from build123d import *

# Parameters (mm, degrees)
SKETCH2_R            = 10
BOSS_EXTRUDE1_DEPTH  = 4
BOSS_EXTRUDE2_DEPTH  = 10
FILLET1_R            = 5
M3_CLEARANCE_HOLE1_D = 3.6
FILLET2_R            = 3


with BuildPart() as part:
    # Sketch2 → Boss-Extrude1 (new body)
    with BuildSketch(Plane(origin=(0, 0, 0), x_dir=(1, 0, 0), z_dir=(0, 1, 0))):
        with BuildLine():
            Line((34.142135624, 5), (34.142135624, -5))
            Line((34.142135624, -5), (14.142135624, -5))
            ThreePointArc((14.142135624, -5), (-15, 0), (14.142135624, 5))
            Line((14.142135624, 5), (34.142135624, 5))
        make_face()
        with Locations(Location((0, 0, 0), (0, 0, 270))):
            Circle(SKETCH2_R, mode=Mode.SUBTRACT)
    extrude(amount=BOSS_EXTRUDE1_DEPTH)

    # Sketch3 → Boss-Extrude2 (add)
    with BuildSketch(Plane.XY.offset(5)):
        Polygon((34.142135624, 4), (34.142135624, 7.343145751), (47.112698372, 20.313708499), (44.284271247, 23.142135624), (30.142135624, 9), (30.142135624, 4), align=None)
    extrude(amount=-BOSS_EXTRUDE2_DEPTH)

    # Fillet1
    fillet1_edges = [part.edges().sort_by_distance(p)[0] for p in [
        (45.69848481, 21.727922061, 5),
        (45.69848481, 21.727922061, -5),
    ]]
    fillet(fillet1_edges, radius=FILLET1_R - 0.0001)  # a hair under: the kernel refuses the full size

    # M3 Clearance Hole1 (through all)
    with Locations(Plane(origin=(10.571067812, -10.571067812, 0), x_dir=(0.7071067811865486, 0.7071067811865466, 0), z_dir=(-0.7071067811865466, 0.7071067811865486, 0))):
        with Locations((42.67766953, 0)):
            Hole(M3_CLEARANCE_HOLE1_D / 2)

    # Fillet2
    fillet2_edges = [part.edges().sort_by_distance(p)[0] for p in [
        (30.142135624, 4, 0),
        (30.142135624, 9, 0),
        (34.142135624, 7.343145751, 0),
        (34.142135624, 0, 0),
    ]]
    fillet(fillet2_edges, radius=FILLET2_R)


solid = part.part
The model under review builds one solid part; all positions refer to its coordinate system, in mm. A direction names the side the tool comes from. Give positions to 0.01 mm unless a question says otherwise; leave off trailing zeros. Order: outer loops, then holes, each group sorted by start corner. A loop starts at its lowest first (then second) coordinate and runs counter-clockwise, first axis right, second up. Notation, with made-up numbers: M 8.5,82.5 L 19.5,82.5 A8 ccw 19.5,97.5 Z; hole C 41,52 d7. An arc over 180 degrees is marked long. Use one line per item in the form item = value. Start each with the question number.
Item 1: We need section C-C on z = -12. Give the boundary of the cut face in (x, y).
Item 2: We need section D-D on x = 36. Give the boundary of the cut face in (y, z).
Item 3: For faces 1 (the flat face through (30, 5, 5)), 2 (the flat face through (34.142, 5, 0)), 3 (the flat face through (14, 0, 0)), 4 (the flat face through (11, 4, 0)), 5 (the cylindrical face through (-9.76, 1.97, -2.17)), list the 3-axis set-ups (+Z, -Z, +X, -X, +Y, -Y) from which the entire face can be reached by the end or side of a thin tool; tool diameter is ignored.
Item 4: We need section A-A on x = 0. Give the boundary of the cut face in (y, z).
Item 5: We need section B-B on z = -6. Give the boundary of the cut face in (x, y).
Item 6: Insertion check: pin 1 Ø12 at (x, y) = (36, 2.5) entering from -Z; pin 2 Ø0.8 at (y, z) = (7.5, -1) entering from -X; pin 3 Ø1.5 at (y, z) = (20, -3.5) entering from -X. Each pin has a flat end and moves straight along its axis. Give the tip position at first contact, or say it passes through.
Item 7: The part is to be moulded in two halves that separate along X. For faces 6 (the cylindrical face through (30.377, 8.921, -0.07)), 7 (the cylindrical face through (43.454, 19.444, -0.079)), 8 (the flat face through (30, 5, -5)), 9 (the cylindrical face through (44.616, 20.685, -3.574)), say which applies: pulls with the +X half, pulls with the -X half, needs draft (parallel to the pull), parting line crosses it, or undercut.
Item 8: To check wall thickness, follow line 1 along X through (y, z) = (2.95, 0); line 2 along X through (y, z) = (3.25, -2); line 3 along Y through (x, z) = (-3, -11.5). State the ranges of each line that lie inside material, in increasing order. Write a range as from..to.
Completed:
q1.outline = M -9,0 L 9,0 L 9,4 L -9,4 Z
q2.outline = M 9.2,-5 L 14.86,-5 L 14.86,5 L 9.2,5 Z
q3.face_1 = +Z, +X, +Y, -Y
q3.face_2 = +Z, -Z, +X, -Y
q3.face_3 = +Z, -Z, +X, -X, -Y
q3.face_4 = +Z, -Z, -X, +Y
q3.face_5 = +Y, -Y
q4.outline = M 0,-15 L 4,-15 L 4,-10 L 0,-10 Z; M 0,10 L 4,10 L 4,15 L 0,15 Z
q5.outline = M -13.75,0 L -8,0 L -8,4 L -13.75,4 Z; M 8,0 L 13.75,0 L 13.75,4 L 8,4 Z
q6.pin_1 = -5
q6.pin_2 = 30.14
q6.pin_3 = 40.39
q7.face_6 = pulls with the -X half
q7.face_7 = undercut
q7.face_8 = needs draft
q7.face_9 = pulls with the +X half
q8.line_1 = -15..-10, 10..34.14
q8.line_2 = -14.87..-9.8, 9.8..34.14
q8.line_3 = 0..4
